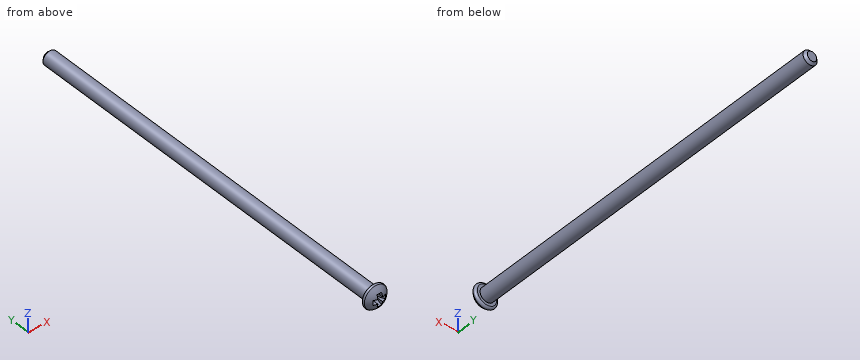
```python
from build123d import *

# Parameters (mm, degrees)
PAD009_DEPTH            = 0.5
BODY005_PLACEMENT_ANGLE = 90
PAD008_DEPTH            = 0.5


with BuildPart() as body005:
    # Sketch021 → Pad009 (new body, symmetric)
    with BuildSketch(Plane.XY):
        Polygon((-2.15, -3.5), (2.15, -3.5), (0.625, 0), (-0.625, 0), align=None)
    extrude(amount=PAD009_DEPTH, both=True)


with BuildPart() as body005_1:
    # Body005 placement: moved
    add(body005.part.rotate(Axis((0, 0, 0), (0, -1, 0)), BODY005_PLACEMENT_ANGLE))


with BuildPart() as fusion:
    # Sketch020 → Pad008 (new body, symmetric)
    with BuildSketch(Plane.XY):
        Polygon((-2.15, -3.5), (2.15, -3.5), (0.625, 0), (-0.625, 0), align=None)
    extrude(amount=PAD008_DEPTH, both=True)

    # Fusion: union Body005
    add(body005_1.part)


with BuildPart() as body007:
    # Sketch019 → Revolution (revolve)
    with BuildSketch(Plane.XY):
        with BuildLine():
            Line((1.5, 0), (1.5, 80.5))
            Line((1.5, 80.5), (1, 81))
            Line((1, 81), (0, 81))
            Line((0, 81), (0, -1.9))
            ThreePointArc((0, -1.9), (1.354762, -1.576681), (2.417511, -0.676413))
            ThreePointArc((2.417511, -0.676413), (2.454213, -0.232991), (2.075154, 0))
            Line((1.5, 0), (2.075154, 0))
        make_face()
    revolve(axis=Axis((0, 0, 0), (0, 1, 0)))

    # Cut: cut Fusion
    add(fusion.part, mode=Mode.SUBTRACT)


with BuildPart() as body007_1:
    # Cut placement: moved
    add(body007.part.moved(Location((-15.9, 3, 25.5))))


with BuildPart() as body007_2:
    # Clone001 placement: moved
    add(body007_1.part.moved(Location((15.9, 0, -25.5))))


with BuildPart() as body007_3:
    # Body007 placement: moved
    add(body007_2.part.moved(Location((-15.9, 0, -25.5))))


solid = body007_3.part
```
Input: part model. Units: mm. Frame: model coordinates. Round coordinates to 2 decimals unless told otherwise and drop trailing zeros. Loops run counter-clockwise (first coordinate to the right, second up) from the corner with the lowest first, then second, coordinate; pieces in that order, holes last.
1) Section query A-A on y = 65. Return the cut outline in (x, z).
Ans:
outline: circle Ø3 at (-15.9, -25.5)
2) Pin query (flat end, axial travel): pin 1 (2 mm diameter, centred on y = 63, z = -23.5, fed in from +X); pin 2 (2 mm diameter, centred on x = -17, y = 74.5, fed in from -Z); pin 3 (0.9 mm diameter, centred on x = -15, y = 2.5, fed in from -Z); pin 4 (2 mm diameter, centred on x = -14.5, z = -25.5, fed in from +Y). Return the tip coordinate at first contact, or that it passes through.
Ans:
pin 1: stops at x = -14.78
pin 2: stops at z = -27
pin 3: stops at z = -27.96
pin 4: stops at y = 84
3) Material intervals for line 1 (X direction, y = 30, z = -25.6); line 2 (Y direction, x = -15.35, z = -25.8); line 3 (Z direction, x = -16.1, y = 50), sorted ascending.
Ans:
line 1: x = -17.4 to -14.4
line 2: y = 3 to 84
line 3: z = -26.99 to -24.01
